```python
from build123d import *

# Parameters (mm, degrees)
CROQUIS1_R              = 11
CROQUIS1_R_2            = 2
CROQUIS1_R_3            = 1.937672591
CROQUIS1_W              = 30
CROQUIS1_H              = 3
SALIENTE_EXTRUIR1_DEPTH = 3
CROQUIS2_R              = 13
CROQUIS2_R_2            = 11
SALIENTE_EXTRUIR2_DEPTH = 4
CROQUIS3_R              = 13
CROQUIS3_R_2            = 9
SALIENTE_EXTRUIR3_DEPTH = 2
CHAFL_N1_SIZE           = 2
CHAFL_N2_SIZE           = 10


with BuildPart() as part:
    # Croquis1 → Saliente-Extruir1 (new body)
    with BuildSketch(Plane(origin=(0, 0, 0), x_dir=(1, 0, 0), z_dir=(0, 1, 0))):
        Polygon((-67.5, 10), (-62.5, 15), (-62.5, -15), (-67.5, -10), (-67.5, -20), (67.5, -20), (67.5, 20), (-67.5, 20), align=None)
        with Locations(Location((46.713951104, 0, 0), (0, 0, 270))):
            Circle(CROQUIS1_R, mode=Mode.SUBTRACT)
        with Locations(Location((-52.5, 0, 0), (0, 0, 270))):
            Circle(CROQUIS1_R_2, mode=Mode.SUBTRACT)
        with Locations(Location((27.185770037, 0, 0), (0, 0, 270))):
            Circle(CROQUIS1_R_3, mode=Mode.SUBTRACT)
        with Locations(Location((12.185770037, 0, 0), (0, 0, 270))):
            Circle(CROQUIS1_R_2, mode=Mode.SUBTRACT)
        with Locations((-27.5, 11)):
            Rectangle(CROQUIS1_W, CROQUIS1_H, mode=Mode.SUBTRACT)
        with Locations((-27.5, -11)):
            Rectangle(CROQUIS1_W, CROQUIS1_H, mode=Mode.SUBTRACT)
    extrude(amount=SALIENTE_EXTRUIR1_DEPTH)

    # Croquis2 → Saliente-Extruir2 (add)
    with BuildSketch(Plane(origin=(0, 3, 0), x_dir=(1, 0, 0), z_dir=(0, 1, 0))):
        with Locations(Location((46.713951104, 0, 0), (0, 0, 90))):
            Circle(CROQUIS2_R)
        with Locations(Location((46.713951104, 0, 0), (0, 0, 270))):
            Circle(CROQUIS2_R_2, mode=Mode.SUBTRACT)
    extrude(amount=SALIENTE_EXTRUIR2_DEPTH)

    # Croquis3 → Saliente-Extruir3 (add)
    with BuildSketch(Plane(origin=(0, 7, 0), x_dir=(1, 0, 0), z_dir=(0, 1, 0))):
        with Locations(Location((46.713951104, 0, 0), (0, 0, 90))):
            Circle(CROQUIS3_R)
        with Locations(Location((46.713951104, 0, 0), (0, 0, 270))):
            Circle(CROQUIS3_R_2, mode=Mode.SUBTRACT)
    extrude(amount=SALIENTE_EXTRUIR3_DEPTH)

    # Chaflán1
    chafl_n1_edges = [part.edges().sort_by_distance(p)[0] for p in [
        (46.713951104, 9, 13),
    ]]
    chamfer(chafl_n1_edges, length=CHAFL_N1_SIZE)

    # Chaflán2
    chafl_n2_edges = [part.edges().sort_by_distance(p)[0] for p in [
        (67.5, 1.5, 20),
        (67.5, 1.5, -20),
    ]]
    chamfer(chafl_n2_edges, length=CHAFL_N2_SIZE)


solid = part.part
```
The listing builds one solid part. Answer for the finished solid, in the listing's coordinates (mm). A direction names the side the tool comes from. Give positions to 0.01 mm unless a question says otherwise; leave off trailing zeros. Write each loop counter-clockwise with the first axis right and the second up, starting at its lowest first coordinate (ties: lowest second). Pieces come first, ordered by that corner, then holes. Notation, with made-up numbers: (35, 41.5) -> (54, 41.5) arc R20 cw to (54, 52.5) -> close; hole circle Ø5 at (-30, 16). An arc over 180 degrees is marked (long way). Write item = value, one per line. Start each with the question number.
1) Determine the mould class of faces 5 (the face through (14.17, 1.48, -0.26)), 6 (the face through (57.62, 3.45, -1.43)), 7 (the face through (62.4, 1.5, 15.1)), 8 (the face through (-4, 1, -20)) for opening direction Z: +Z half, -Z half, draft (parallel to the pull), parting line (faces both ways), or undercut.
2) The part is cut by section C-C, the plane x = -15. Determine the outline of the cut face in (y, z).
3) Which of the six approach directions +Z, -Z, +X, -X, +Y, -Y give full straight-line access (tool end or side, diameter ignored) to faces 1 (the face through (55, 7, 4)), 2 (the face through (62.6, 1.5, -14.9)), 3 (the face through (59.405, 4.972, 2.818)), 4 (the face through (-28, 1, -9.5))?
4) The part is cut by section A-A, the plane x = -52.5. Determine the outline of the cut face in (y, z), and give its area (3 significant figures).
5) The part is cut by section B-B, the plane z = 0. Count the separate pieces of the cut face and the enclosed holes in it, and give its area (3 significant figures).
6) Each of these flat-tipped pins is pushed along its axis until it touches: pin 1 (14.5 mm diameter, centred on x = 46.71, z = 0, fed in from -Y); pin 2 (0.9 mm diameter, centred on y = 1, z = -11, fed in from +X); pin 3 (0.9 mm diameter, centred on y = 1.5, z = -3, fed in from -X); pin 4 (5 mm diameter, centred on x = -33.5, z = -2, fed in from +Y). Where does it stop, or does it pass through?
7) Straight lines are drawn through the part: line 1 along X through (y, z) = (0.8, 0); line 2 along Y through (x, z) = (-55, -8); line 3 along X through (y, z) = (5.5, -5.5). For each, find the intervals that lie inside material, in ascending order.
8) The part is cut by section D-D, the plane y = 4.5. Determine the outline of the cut face in (x, z), and give its area (3 significant figures).
Solutions:
q1.face_5 = undercut
q1.face_6 = undercut
q1.face_7 = +Z half
q1.face_8 = -Z half
q2.outline = (0, -20) -> (3, -20) -> (3, -12.5) -> (0, -12.5) -> close; (0, -9.5) -> (3, -9.5) -> (3, 9.5) -> (0, 9.5) -> close; (0, 12.5) -> (3, 12.5) -> (3, 20) -> (0, 20) -> close
q3.face_1 = -Y
q3.face_2 = -Z, +X, +Y, -Y
q3.face_3 = +Y
q3.face_4 = +Y, -Y
q4.outline = (0, -20) -> (3, -20) -> (3, -2) -> (0, -2) -> close; (0, 2) -> (3, 2) -> (3, 20) -> (0, 20) -> close
q4.area = 108 mm²
q5.separate_pieces = 5
q5.enclosed_holes = 0
q5.area = 316 mm²
q6.pin_1 = through
q6.pin_2 = 66.95
q6.pin_3 = -62.5
q6.pin_4 = 3
q7.line_1 = -62.5 to -54.5, -50.5 to 10.19, 14.19 to 25.25, 29.12 to 35.71, 57.71 to 67.5
q7.line_2 = 0 to 3
q7.line_3 = 34.93 to 37.19, 56.24 to 58.49
q8.outline = circle Ø26 at (46.71, 0); hole circle Ø22 at (46.71, 0)
q8.area = 151 mm²
